Print and shaded views of the part. All mm, measured from the part's lowest x, y and z. A direction names the side the tool comes from. Coordinates: 2 decimals unless noted, no trailing zeros. Order: outer loops, then holes, each group sorted by start corner. A loop starts at its lowest first (then second) coordinate and runs counter-clockwise, first axis right, second up. Notation, with made-up numbers: M 35.5,67.25 L 78.5,67.25 A8 cw 78.5,82.25 Z; hole C 71,-24 d4. An arc over 180 degrees is marked long. One line per item, written item: value.
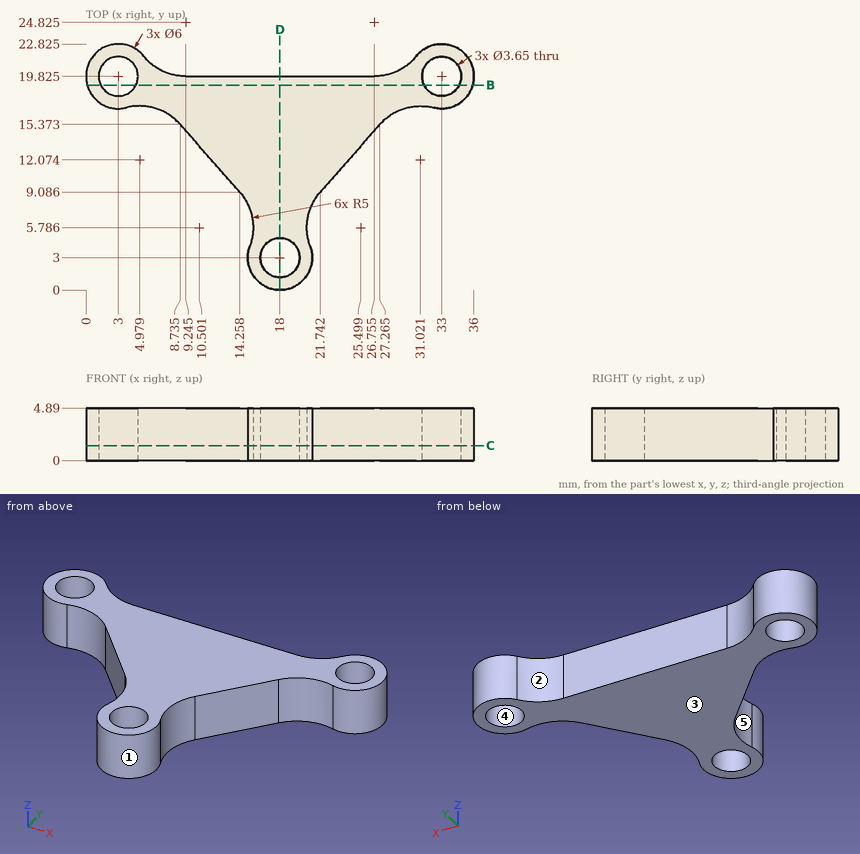
Q1. Slice it at D-D (x = 18). List the corners of the cut face in (y, z) (1 decimal).
Recorded:
outline: M 0,0 L 1.2,0 L 1.2,4.9 L 0,4.9 Z; M 4.8,0 L 19.8,0 L 19.8,4.9 L 4.8,4.9 Z
Q2. Drill centre lines: line 1 along X through (y, z) = (3, 3.45) (1 decimal); line 2 along X through (y, z) = (19.5, 0.4) (1 decimal); line 3 along Y through (x, z) = (18, 1.3) (1 decimal). Where is each one in solid material? Low to high.
Recorded:
line 1: x = 15 to 16.2, 19.8 to 21
line 2: x = 0 to 1.2, 4.8 to 31.2, 34.8 to 36
line 3: y = 0 to 1.2, 4.8 to 19.8
Q3. Mould opens along X. For the marked faces 3, 4 and 5 say: released by +X, released by -X, zero draft, split by the parting line, or undercut.
Recorded:
face 3: zero draft
face 4: undercut
face 5: released by -X
Q4. Slice it at B-B (y = 19). List the corners of the cut face in (x, z) (1 decimal).
Recorded:
outline: M 0.1,0 L 1.4,0 L 1.4,4.9 L 0.1,4.9 Z; M 4.6,0 L 31.4,0 L 31.4,4.9 L 4.6,4.9 Z; M 34.6,0 L 35.9,0 L 35.9,4.9 L 34.6,4.9 Z
Q5. Which spindle directions (+Z, -Z, +X, -X, +Y, -Y) get a long thin tool onto all of the face, cutting with end or side? Do the marked faces 1 and 2. Say none if no direction does.
Recorded:
face 1: +Z, -Z
face 2: +Z, -Z, +Y
Q6. Pin check, flat tips, straight feed: pin 1 Ø3 at (x, y) = (18, 3) entering from +Z; pin 2 Ø2.5 at (x, z) = (16.5, 2) entering from +Y (3 decimals). Stop position of each tip, or through.
Recorded:
pin 1: passes through
pin 2: stops at y = 19.825
Q7. Slice it at C-C (z = 1.4). Give the number of separate pieces and of enclosed holes in the cut face.
Recorded:
separate pieces: 1
enclosed holes: 3
